from build123d import *

# Parameters (mm, degrees)
F0_W     = 120
F0_H     = 10
F1_DEPTH = 80
F3_DEPTH = 80.001
F4_DEPTH = 25
F5_W     = 10
F5_H     = 10
F6_DEPTH = 70.001


with BuildPart() as f1:
    # F0 (on Right) → F1 (new body)
    with BuildSketch(Plane.YZ):
        Rectangle(F0_W, F0_H)
        with BuildLine():
            ThreePointArc((60, 5), (0, 65), (-60, 5))
            Line((-60, 5), (60, 5))
        make_face()
    extrude(amount=F1_DEPTH)

    # F2 (on face) → F3 (cut, through all)
    with BuildSketch(Plane.YZ.offset(80)):
        with BuildLine():
            Line((-5, 5), (5, 5))
            ThreePointArc((5, 5), (0, 10), (-5, 5))
        make_face()
        with BuildLine():
            ThreePointArc((-5, 5), (0, 0), (5, 5))
            Line((5, 5), (-5, 5))
        make_face()
        with BuildLine():
            ThreePointArc((-5, 5), (0, 10), (5, 5))
            Line((5, 5), (35, 5))
            ThreePointArc((35, 5), (36.3556550657, 8.4232659844), (39.6875, 9.9902248196))
            ThreePointArc((39.6875, 9.9902248196), (0, 45), (-39.6875, 9.9902248196))
            ThreePointArc((-39.6875, 9.9902248196), (-36.3556550657, 8.4232659844), (-35, 5))
            Line((-35, 5), (-5, 5))
        make_face()
        with BuildLine():
            Line((40, 5), (35, 5))
            ThreePointArc((35, 5), (40, 0), (45, 5))
            ThreePointArc((45, 5), (43.4232659844, 8.6443449343), (39.6875, 9.9902248196))
            ThreePointArc((39.6875, 9.9902248196), (39.9217985567, 7.5), (40, 5))
        make_face()
        with BuildLine():
            ThreePointArc((39.6875, 9.9902248196), (36.3556550657, 8.4232659844), (35, 5))
            Line((35, 5), (40, 5))
            ThreePointArc((40, 5), (39.9217985567, 7.5), (39.6875, 9.9902248196))
        make_face()
        with BuildLine():
            Line((-40, 5), (-35, 5))
            ThreePointArc((-35, 5), (-36.3556550657, 8.4232659844), (-39.6875, 9.9902248196))
            ThreePointArc((-39.6875, 9.9902248196), (-39.9217985567, 7.5), (-40, 5))
        make_face()
        with BuildLine():
            ThreePointArc((-39.6875, 9.9902248196), (-43.6443449343, 1.5767340156), (-35, 5))
            Line((-35, 5), (-40, 5))
            ThreePointArc((-40, 5), (-39.9217985567, 7.5), (-39.6875, 9.9902248196))
        make_face()
    extrude(amount=-F3_DEPTH, mode=Mode.SUBTRACT)

    # F2 (on face) → F4 (cut)
    with BuildSketch(Plane.YZ.offset(80)):
        with BuildLine():
            Line((-5, 5), (5, 5))
            ThreePointArc((5, 5), (0, 10), (-5, 5))
        make_face()
        with BuildLine():
            ThreePointArc((-5, 5), (0, 0), (5, 5))
            Line((5, 5), (-5, 5))
        make_face()
        with BuildLine():
            ThreePointArc((-5, 5), (0, 10), (5, 5))
            Line((5, 5), (35, 5))
            ThreePointArc((35, 5), (36.3556550657, 8.4232659844), (39.6875, 9.9902248196))
            ThreePointArc((39.6875, 9.9902248196), (0, 45), (-39.6875, 9.9902248196))
            ThreePointArc((-39.6875, 9.9902248196), (-36.3556550657, 8.4232659844), (-35, 5))
            Line((-35, 5), (-5, 5))
        make_face()
        with BuildLine():
            Line((40, 5), (35, 5))
            ThreePointArc((35, 5), (40, 0), (45, 5))
            ThreePointArc((45, 5), (43.4232659844, 8.6443449343), (39.6875, 9.9902248196))
            ThreePointArc((39.6875, 9.9902248196), (39.9217985567, 7.5), (40, 5))
        make_face()
        with BuildLine():
            ThreePointArc((39.6875, 9.9902248196), (36.3556550657, 8.4232659844), (35, 5))
            Line((35, 5), (40, 5))
            ThreePointArc((40, 5), (39.9217985567, 7.5), (39.6875, 9.9902248196))
        make_face()
        with BuildLine():
            Line((-40, 5), (-35, 5))
            ThreePointArc((-35, 5), (-36.3556550657, 8.4232659844), (-39.6875, 9.9902248196))
            ThreePointArc((-39.6875, 9.9902248196), (-39.9217985567, 7.5), (-40, 5))
        make_face()
        with BuildLine():
            ThreePointArc((-39.6875, 9.9902248196), (-43.6443449343, 1.5767340156), (-35, 5))
            Line((-35, 5), (-40, 5))
            ThreePointArc((-40, 5), (-39.9217985567, 7.5), (-39.6875, 9.9902248196))
        make_face()
    extrude(amount=-F4_DEPTH, mode=Mode.SUBTRACT)

    # F5 (on face) → F6 (cut, through all)
    with BuildSketch(Plane(origin=(0, 0, -5), x_dir=(1, 0, 0), z_dir=(0, 0, -1))):
        with Locations((40, 45.0840815902)):
            Rectangle(F5_W, F5_H)
        with Locations((40, 0)):
            Rectangle(F5_W, F5_H)
        with Locations((40, -48.8508976996)):
            Rectangle(F5_W, F5_H)
    extrude(amount=-F6_DEPTH, mode=Mode.SUBTRACT)


solid = f1.part
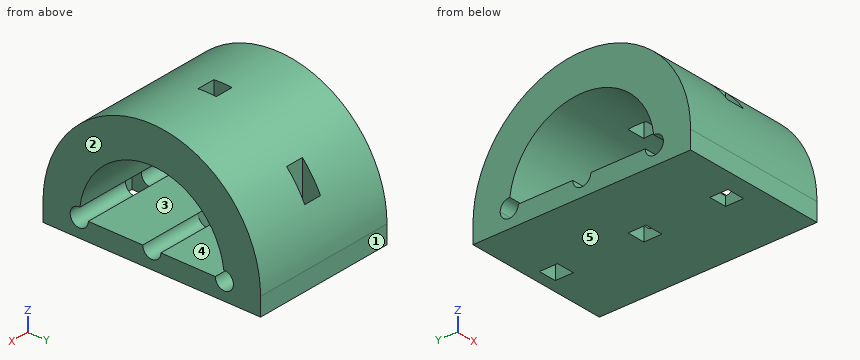
Build history of the part. All positions in model axes, mm. Face numbers are marked on the shaded views. A direction names the side the tool comes from. Round coordinates to 2 decimals unless told otherwise and drop trailing zeros. Loops run counter-clockwise (first coordinate to the right, second up) from the corner with the lowest first, then second, coordinate; pieces in that order, holes last. Notation, with made-up numbers: (52, 44) -> (85, 44) arc R32 cw to (85, 76) -> close; hole circle Ø2 at (73.5, 69.5). An arc over 180 degrees is marked (long way). Use CSV: the item, a comma, the result in double quotes. Start each with the question number.
Q1. Drill centre lines: L1, parallel to Y at x = 40.5, z = 24; L2, parallel to Y at x = 47, z = 2.5; L3, parallel to X at y = 52.5, z = 13.5. Where is each one in solid material? Low to high.
Q2. Which spindle directions (+Z, -Z, +X, -X, +Y, -Y) get a long thin tool onto all of the face, cutting with end or side? Do the marked faces 4 and 5. Say none if no direction does.
Q3. Saw through at A-A on x = 42.5. Give the cut face in (y, z).
Q4. Saw through at C-C on z = 33. Give the cut face in (x, y).
Q5. Saw through at D-D on y = -32. Give the cut face in (x, z).
Q6. Saw through at B-B on y = 0. Give the cut face in (x, z), and give its area (3 significant figures).
Q7. Flat gauge pins, fed straight in: pin 1 Ø3 at (y, z) = (46.5, 15.5) entering from -X; pin 2 Ø11 at (x, z) = (40.5, 22.5) entering from -Y; pin 3 Ø8 at (x, z) = (42, 50.5) entering from -Y; pin 4 Ø1 at (x, z) = (55, 26.5) entering from -Y (3 decimals). Where does each tip first touch, or does it go through?
Q8. Mould opens along Y. For the marked faces 1, 2 and 3 say: +Y half, -Y half, draft (parallel to the pull), parting line (faces both ways), or undercut.
Solutions:
1,L1,"y = -56.91 to -50.08, -40.08 to -35.2, 35.2 to 43.85, 53.85 to 56.91"
1,L2,"y = -60 to -44.33, -35.67 to -4.33, 4.33 to 35.67, 44.33 to 60"
1,L3,"x = 0 to 35, 45 to 80"
2,face 4,"+X, -X"
2,face 5,"-Z, +X, -X, +Y, -Y"
3,outline,"(-60, -5) -> (-50.08, -5) -> (-50.08, 38.04) arc R60 ccw to (-60, 5) -> close; (-40.08, -5) -> (-5, -5) -> (-5, 5) -> (-35, 5) arc R5 cw to (-40.08, 0) -> close; (-40.08, 10) arc R5 cw to (-39.69, 9.99) arc R40 cw to (-5, 44.69) -> (-5, 64.79) arc R60 ccw to (-40.08, 49.65) -> close; (5, -5) -> (43.85, -5) -> (43.85, 1.81) arc R5 cw to (35, 5) -> (5, 5) -> close; (5, 44.69) arc R40 cw to (39.69, 9.99) arc R5 cw to (43.85, 8.19) -> (43.85, 45.95) arc R60 ccw to (5, 64.79) -> close; (53.85, -5) -> (60, -5) -> (60, 5) arc R60 ccw to (53.85, 31.46) -> close"
4,outline,"(0, -53.07) -> (80, -53.07) -> (80, -28.57) -> (0, -28.57) -> close; (0, 28.57) -> (80, 28.57) -> (80, 53.07) -> (45, 53.07) -> (45, 43.85) -> (35, 43.85) -> (35, 53.07) -> (0, 53.07) -> close; hole (35, -50.08) -> (45, -50.08) -> (45, -40.08) -> (35, -40.08) -> close"
5,outline,"(0, -5) -> (80, -5) -> (80, 5) -> (0, 5) -> close; (0, 29) -> (80, 29) -> (80, 55.75) -> (0, 55.75) -> close"
6,outline,"(0, -5) -> (35, -5) -> (35, 0) -> (0, 0) -> close; (0, 45) -> (35, 45) -> (35, 65) -> (0, 65) -> close; (45, -5) -> (80, -5) -> (80, 0) -> (45, 0) -> close; (45, 45) -> (80, 45) -> (80, 65) -> (45, 65) -> close"
6,area,"1,750 mm^2"
7,pin 1,"stops at x = 0"
7,pin 2,"stops at y = -58.79"
7,pin 3,"stops at y = -41.99"
7,pin 4,"stops at y = -56.205"
8,face 1,"+Y half"
8,face 2,"draft"
8,face 3,"undercut"
